Geometry check sheet. Reference: the model listing, model coordinates, mm. A direction names the side the tool comes from. Give positions to 0.01 mm unless a question says otherwise; leave off trailing zeros. Order: outer loops, then holes, each group sorted by start corner. A loop starts at its lowest first (then second) coordinate and runs counter-clockwise, first axis right, second up. Notation, with made-up numbers: M 86.25,48.25 L 118.25,48.25 A24 cw 118.25,79.25 Z; hole C -3.5,38.5 d10. An arc over 180 degrees is marked long. Answer as CSV lines item,"result".
from build123d import *

# Parameters (mm, degrees)
F0_W         = 55.88
F0_H         = 25.4
F1_DEPTH     = 13.716
F2_W         = 20.32
F2_H         = 8.89
F3_DEPTH     = 13.717
F4_W         = 20.32
F4_H         = 8.89
F5_DEPTH     = 13.717
F6_W         = 15.24
F6_H         = 3.937
F7_DEPTH     = 7.366
F8_W         = 15.24
F8_H         = 3.937
F9_DEPTH     = 7.366
F10_W        = 55.88
F10_H        = 18.796
F11_DEPTH    = 9.398
F12_W        = 20.32
F12_H        = 6.858
F13_DEPTH    = 25.401
F14_W        = 20.32
F14_H        = 6.858
F15_DEPTH    = 25.401
F17_DEPTH    = 25.401
F19_DEPTH    = 25.401
F20_R        = 1.27
F21_W        = 38.1
F21_H        = 20.955
F22_DEPTH    = 9.398
F23_W        = 38.1
F23_H        = 20.955
F24_DEPTH    = 9.398
F25_T1_DEPTH = 28.8734423739
F26_W        = 1.778
F26_H        = 20.955
F27_DEPTH    = 2.54
F28_W        = 1.778
F28_H        = 20.955
F29_DEPTH    = 2.54
F30_W        = 55.88
F30_H        = 12.7
F31_DEPTH    = 2.54
F32_SIZE     = 3.81
F33_R        = 0.635


# Not quite as in the source:
# - a fillet or chamfer that OpenCascade refuses, or shapes differently, is made with other operations: its cross-section is extruded or revolved along the edge and cut away or added


with BuildPart() as f1:
    # F0 (on Top) → F1 (new body)
    with BuildSketch(Plane.XY):
        Rectangle(F0_W, F0_H)
    extrude(amount=F1_DEPTH)

    # F2 (on face) → F3 (cut, through all)
    with BuildSketch(Plane(origin=(0, 0, 0), x_dir=(1, 0, 0), z_dir=(0, 0, -1))):
        with Locations((17.78, 0)):
            Rectangle(F2_W, F2_H)
    extrude(amount=-F3_DEPTH, mode=Mode.SUBTRACT)

    # F4 (on face) → F5 (cut, through all)
    with BuildSketch(Plane(origin=(0, 0, 0), x_dir=(1, 0, 0), z_dir=(0, 0, -1))):
        with Locations((-17.78, 0)):
            Rectangle(F4_W, F4_H)
    extrude(amount=-F5_DEPTH, mode=Mode.SUBTRACT)

    # F6 (on face) → F7 (cut)
    with BuildSketch(Plane(origin=(0, 0, 0), x_dir=(1, 0, 0), z_dir=(0, 0, -1))):
        with Locations((0, 8.4455)):
            Rectangle(F6_W, F6_H)
    extrude(amount=-F7_DEPTH, mode=Mode.SUBTRACT)

    # F8 (on face) → F9 (cut)
    with BuildSketch(Plane(origin=(0, 0, 0), x_dir=(1, 0, 0), z_dir=(0, 0, -1))):
        with Locations((0, -8.4455)):
            Rectangle(F8_W, F8_H)
    extrude(amount=-F9_DEPTH, mode=Mode.SUBTRACT)

    # F10 (on face) → F11 (cut)
    with BuildSketch(Plane.XY.offset(13.716)):
        Rectangle(F10_W, F10_H)
    extrude(amount=-F11_DEPTH, mode=Mode.SUBTRACT)

    # F12 (on face) → F13 (cut, through all)
    with BuildSketch(Plane.XZ.offset(12.7)):
        with Locations((-12.7, 10.287)):
            Rectangle(F12_W, F12_H)
    extrude(amount=-F13_DEPTH, mode=Mode.SUBTRACT)

    # F14 (on face) → F15 (cut, through all)
    with BuildSketch(Plane.XZ.offset(12.7)):
        with Locations((12.7, 10.287)):
            Rectangle(F14_W, F14_H)
    extrude(amount=-F15_DEPTH, mode=Mode.SUBTRACT)

    # F16 (on face) → F17 (cut, through all)
    with BuildSketch(Plane.XZ.offset(12.7)):
        Polygon((-25.4, 13.716), (-22.86, 6.858), (-22.86, 13.716), align=None)
    extrude(amount=-F17_DEPTH, mode=Mode.SUBTRACT)

    # F18 (on face) → F19 (cut, through all)
    with BuildSketch(Plane.XZ.offset(12.7)):
        Polygon((22.86, 13.716), (22.86, 6.858), (25.4, 13.716), align=None)
    extrude(amount=-F19_DEPTH, mode=Mode.SUBTRACT)

    # F20
    f20_edges = [f1.edges().sort_by_distance(p)[0] for p in [
        (-25.4, 11.049, 13.716),
        (-25.4, -11.049, 13.716),
        (25.4, 11.049, 13.716),
        (25.4, -11.049, 13.716),
        (-27.94, 11.049, 13.716),
        (-27.94, -11.049, 13.716),
        (27.94, -11.049, 13.716),
        (27.94, 11.049, 13.716),
    ]]
    fillet(f20_edges, radius=F20_R)

    # F21 (on face) → F22 (cut)
    with BuildSketch(Plane.XY.offset(13.716)):
        with Locations((-21.6148423028, 0)):
            Rectangle(F21_W, F21_H)
    extrude(amount=-F22_DEPTH, mode=Mode.SUBTRACT)

    # F23 (on face) → F24 (cut)
    with BuildSketch(Plane.XY.offset(13.716)):
        with Locations((21.6445253996, 0)):
            Rectangle(F23_W, F23_H)
    extrude(amount=-F24_DEPTH, mode=Mode.SUBTRACT)

    # F25: fillet of radius 5.08 on 2 edges, made by hand

    # F25_s2 → F25_t1 (cut)
    with BuildSketch(Plane.YZ.offset(-14.4367211869)):
        with BuildLine():
            ThreePointArc((9.398, 8.9573115252), (10.3043541118, 11.853357105), (12.7, 13.716))
            Line((12.7, 13.716), (9.398, 13.716))
            Line((9.398, 13.716), (9.398, 8.9573115252))
        make_face()
        with BuildLine():
            ThreePointArc((-12.7, 13.716), (-10.3043541118, 11.853357105), (-9.398, 8.9573115252))
            Line((-9.398, 8.9573115252), (-9.398, 13.716))
            Line((-9.398, 13.716), (-12.7, 13.716))
        make_face()
    extrude(amount=F25_T1_DEPTH, mode=Mode.SUBTRACT)

    # F26 (on face) → F27 (join)
    with BuildSketch(Plane.XY.offset(4.318)):
        with Locations((21.209, 0)):
            Rectangle(F26_W, F26_H)
    extrude(amount=F27_DEPTH)

    # F28 (on face) → F29 (join)
    with BuildSketch(Plane.XY.offset(4.318)):
        with Locations((-21.209, 0)):
            Rectangle(F28_W, F28_H)
    extrude(amount=F29_DEPTH)

    # F30 (on face) → F31 (cut)
    with BuildSketch(Plane.XY.offset(6.858)):
        with Locations((-0.1600864343, 0)):
            Rectangle(F30_W, F30_H)
    extrude(amount=-F31_DEPTH, mode=Mode.SUBTRACT)

    # F32
    f32_edges = [f1.edges().sort_by_distance(p)[0] for p in [
        (7.62, 0, 4.318),
        (-7.62, 0, 4.318),
    ]]
    chamfer(f32_edges, length=F32_SIZE)

    # F33
    f33_edges = [f1.edges().sort_by_distance(p)[0] for p in [
        (27.94, -12.7, 6.223),
        (27.568026, -12.7, 13.344026),
        (0, -12.7, 0),
        (26.476968, -12.7, 13.716),
        (-27.94, -12.7, 6.223),
        (25.558431, -12.7, 13.488373),
        (-27.568026, -12.7, 13.344026),
        (23.976498, -12.7, 9.872545),
        (-26.476968, -12.7, 13.716),
        (12.7, -12.7, 6.858),
        (-25.558431, -12.7, 13.488373),
        (2.54, -12.7, 10.287),
        (-23.976498, -12.7, 9.872545),
        (0, -12.7, 13.716),
        (-12.7, -12.7, 6.858),
        (-2.54, -12.7, 10.287),
        (-27.94, 12.7, 6.223),
        (-27.568026, 12.7, 13.344026),
        (0, 12.7, 0),
        (-26.476968, 12.7, 13.716),
        (27.94, 12.7, 6.223),
        (-25.558431, 12.7, 13.488373),
        (27.568026, 12.7, 13.344026),
        (-23.976498, 12.7, 9.872545),
        (26.476968, 12.7, 13.716),
        (-12.7, 12.7, 6.858),
        (25.558431, 12.7, 13.488373),
        (-2.54, 12.7, 10.287),
        (23.976498, 12.7, 9.872545),
        (0, 12.7, 13.716),
        (12.7, 12.7, 6.858),
        (2.54, 12.7, 10.287),
    ]]
    fillet(f33_edges, radius=F33_R)


solid = f1.part
(1) Material ranges on line 1 (X direction, y = 10, z = 1.75); line 2 (Y direction, x = -7.5, z = 4.5); line 3 (Y direction, x = 9, z = 1) (3 decimals), recorded low to high.
The answers:
line 1,"x = -27.94 to -7.62, 7.62 to 27.94"
line 2,"y = -12.7 to -10.48, 10.48 to 12.7"
line 3,"y = -12.7 to -4.445, 4.445 to 12.7"
(2) Section check B-B on x = 11. Enter the section's corners in (y, z) (1 decimal).
The answers:
outline,"M -12.7,0.6 A0.6 ccw -12.1,0 L -4.4,0 L -4.4,4.3 L -10.5,4.3 L -10.5,6.9 L -12.1,6.9 A0.6 ccw -12.7,6.2 Z; M 4.4,0 L 12.1,0 A0.6 ccw 12.7,0.6 L 12.7,6.2 A0.6 ccw 12.1,6.9 L 10.5,6.9 L 10.5,4.3 L 4.4,4.3 Z"
(3) Section check C-C on x = -7. State how many separate pieces and enclosed holes the cut face has, then the cut area to 3 significant figures.
The answers:
separate pieces,"3"
enclosed holes,"0"
area,"58.3 mm2"
(4) Section check A-A on y = 7.75. Enter the section's corners in (x, z).
The answers:
outline,"M -27.94,0 L -7.62,0 L -7.62,4.32 L -20.32,4.32 L -20.32,6.86 L -22.1,6.86 L -22.1,4.32 L -27.94,4.32 Z; M 7.62,0 L 27.94,0 L 27.94,4.32 L 22.1,4.32 L 22.1,6.86 L 20.32,6.86 L 20.32,4.32 L 7.62,4.32 Z"
(5) Section check D-D on z = 2.75. Enter the section's corners in (x, y) (3 decimals), then the cut area to 3 significant figures.
The answers:
outline,"M -27.94,-12.065 A0.635 ccw -27.305,-12.7 L 27.305,-12.7 A0.635 ccw 27.94,-12.065 L 27.94,-4.445 L 5.378,-4.445 L 5.378,4.445 L 27.94,4.445 L 27.94,12.065 A0.635 ccw 27.305,12.7 L -27.305,12.7 A0.635 ccw -27.94,12.065 L -27.94,4.445 L -5.378,4.445 L -5.378,-4.445 L -27.94,-4.445 Z; hole M -7.62,-10.414 L 7.62,-10.414 L 7.62,-6.477 L -7.62,-6.477 Z; hole M -7.62,6.477 L 7.62,6.477 L 7.62,10.414 L -7.62,10.414 Z"
area,"898 mm2"
(6) Draft check along X on faces 1 (the face through (0, 10, 7.366)), 2 (the face through (27.58, 11.28, 13.33)), 3 (the face through (2.54, -11, 10)). Enter one of: +X half, -X half, draft (parallel to the pull), parting line (faces both ways), or undercut.
The answers:
face 1,"draft"
face 2,"+X half"
face 3,"undercut"
(7) Gauge pin test, flat ends, axial feed: P1, Ø4.5, axis at x = 15, y = -9.5, coming from the +Z side; P2, Ø5, axis at x = -16, y = -6, coming from the +Z side; P3, Ø1.3, axis at y = -8.5, z = 6, coming from the -X side. Record the tip position at first contact, or that the pin passes through.
The answers:
P1,"stops at z = 6.86"
P2,"stops at z = 4.32"
P3,"stops at x = -22.1"
(8) Tool access check on faces 4 (the face through (-24.06, 12.52, 9.55)), 5 (the face through (21, -6.35, 6)), 6 (the face through (-14, -11, 6.858)), 7 (the face through (22.098, 8, 6)), 8 (the face through (0, 6.477, 2)). Record the directions out of +Z, -Z, +X, -X, +Y, -Y that give a thin tool (end or side, any length) a straight path to the whole face; none if there is none.
The answers:
face 4,"+Z, +Y"
face 5,"+Z, +X, -X"
face 6,"+Z, +Y, -Y"
face 7,"+Z, +X"
face 8,"+Z, -Z"
